For this review, use the dimensioned drawing (mm, ordinates from the lowest corner) and the shaded views. Coordinates: 2 decimals unless noted, no trailing zeros. Order: outer loops, then holes, each group sorted by start corner. A loop starts at its lowest first (then second) coordinate and runs counter-clockwise, first axis right, second up. Notation, with made-up numbers: M -10.75,85.5 L 47.25,85.5 A19 ccw 47.25,89.5 Z; hole C 24.5,13.25 d10. An arc over 180 degrees is marked long. Answer in a Markdown table with one row per item.
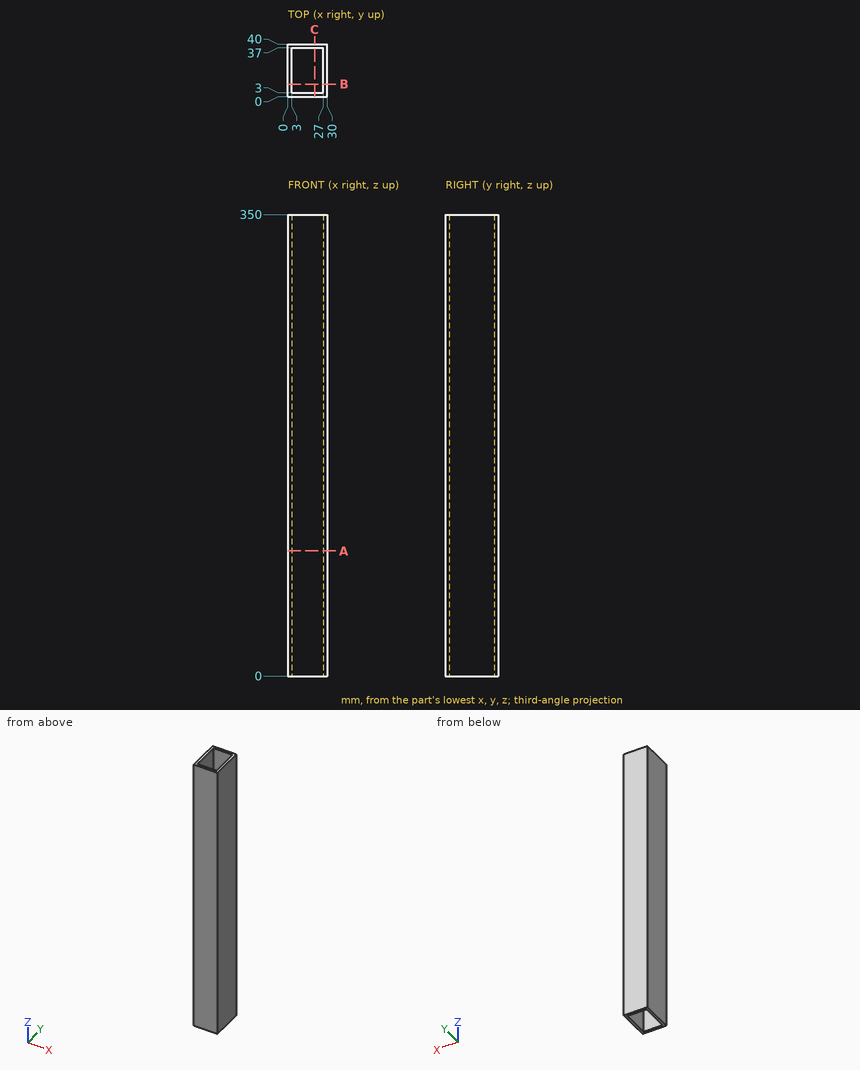
(1) Add section B-B, the plane y = 9.5. Give the boundary of the cut face in (x, z), and give its area (3 significant figures).
Return value:
| item | result |
|---|---|
| outline | M 0,0 L 3,0 L 3,350 L 0,350 Z; M 27,0 L 30,0 L 30,350 L 27,350 Z |
| area | 2,100 mm2 |
(2) Add section C-C, the plane x = 20.25. Give the boundary of the cut face in (y, z), and give its area (3 significant figures).
Return value:
| item | result |
|---|---|
| outline | M 0,0 L 3,0 L 3,350 L 0,350 Z; M 37,0 L 40,0 L 40,350 L 37,350 Z |
| area | 2,100 mm2 |
(3) Add section A-A, the plane z = 95. Give the boundary of the cut face in (x, y).
Return value:
| item | result |
|---|---|
| outline | M 0,0 L 30,0 L 30,40 L 0,40 Z; hole M 3,3 L 27,3 L 27,37 L 3,37 Z |
(4) For line 1 along Y through (x, z) = (15.5, 89.5); line 2 along X through (y, z) = (5.5, 129), list the stretches that pass through material, from the lowest coordinate up. Write a range as from..to.
Return value:
| item | result |
|---|---|
| line 1 | y = 0..3, 37..40 |
| line 2 | x = 0..3, 27..30 |
